Read the model definition and answer for the solid it produces. Units are mm, in the model's axes. Give positions to 0.01 mm unless a question says otherwise; leave off trailing zeros. Loops run counter-clockwise (first coordinate to the right, second up) from the corner with the lowest first, then second, coordinate; pieces in that order, holes last. Notation, with made-up numbers: (-10, 29.5) - (10, 29.5) arc R14 ccw to (10, 40.5) - close; hole circle Ø9 at (87.5, 47.25). An arc over 180 degrees is marked (long way). Use a Markdown table: item, result. Add a question column.
Item 1: A cutting plane is placed at A-A (x = 2.5). Determine the outline of the cut face in (y, z) (3 decimals), plus the area to 3 significant figures.
Item 2: A cutting plane is placed at C-C (z = 11.5). Determine the outline of the cut face in (x, y).
Item 3: This flat-tipped pin is pushed along its axis until it touches: P1, Ø3, axis at x = 3.175, z = -26.843, coming from the -Y side. Where does it stop, or does it pass through?
Item 4: A cutting plane is placed at B-B (y = 10). Give the number of separate pieces and of enclosed holes in the cut face, plus the area to 3 significant figures.
Item 5: Consider probe 1 along Z at (x, y) = (5.25, 3) (3 decimals); probe 2 along X at (y, z) = (11, -26.5); probe 3 along Z at (x, y) = (1, 5) (3 decimals). Determine where each line is inside the solid, lowest interval first. Write a range as [from, to].
from build123d import *

# Parameters (mm, degrees)
BOSS_EXTRUDE2_DEPTH = 6.35
SKETCH8_R           = 2.38125
CUT_EXTRUDE3_DEPTH  = 12.7


with BuildPart() as part:
    # Sketch7 → Boss-Extrude2 (new body)
    with BuildSketch(Plane(origin=(0, 0, 0), x_dir=(0, 0, -1), z_dir=(1, 0, 0))):
        Polygon((211.186, 0), (0, 0), (-37.279, 0), (-37.279, 5.533348483), (5.116676416, 12.7), (206.069323584, 12.7), (248.465, 5.533348483), (248.465, 0), align=None)
    extrude(amount=BOSS_EXTRUDE2_DEPTH)

    # Sketch8 → Cut-Extrude3 (cut)
    with BuildSketch(Plane.XZ):
        with Locations((3.175, -26.843)):
            Circle(SKETCH8_R)
        with Locations((3.175, -79.343)):
            Circle(SKETCH8_R)
        with Locations((3.175, -131.843)):
            Circle(SKETCH8_R)
        with Locations((3.175, -184.343)):
            Circle(SKETCH8_R)
    extrude(amount=-CUT_EXTRUDE3_DEPTH, mode=Mode.SUBTRACT)


solid = part.part
Geometry says:
| question | item | result |
|---|---|---|
| 1 | outline | (0, -248.465) - (5.533, -248.465) - (12.7, -206.069) - (12.7, -186.627) - (0, -186.627) - close; (0, -182.059) - (12.7, -182.059) - (12.7, -134.127) - (0, -134.127) - close; (0, -129.559) - (12.7, -129.559) - (12.7, -81.627) - (0, -81.627) - close; (0, -77.059) - (12.7, -77.059) - (12.7, -29.127) - (0, -29.127) - close; (0, -24.559) - (12.7, -24.559) - (12.7, -5.117) - (5.533, 37.279) - (0, 37.279) - close |
| 1 | area | 3,090 mm² |
| 2 | outline | (0, 0) - (6.35, 0) - (6.35, 9.89) - (0, 9.89) - close |
| 3 | P1 | through |
| 4 | separate pieces | 1 |
| 4 | enclosed holes | 4 |
| 4 | area | 1,410 mm² |
| 5 | probe 1 | [-248.465, -185.511], [-183.175, -133.011], [-130.675, -80.511], [-78.175, -28.011], [-25.675, 37.279] |
| 5 | probe 2 | [0, 0.82], [5.53, 6.35] |
| 5 | probe 3 | [-248.465, -185.312], [-183.374, -132.812], [-130.874, -80.312], [-78.374, -27.812], [-25.874, 37.279] |
